Can you work these out from the model? Positions are in its coordinate system, mm. Give positions to 0.01 mm unless a question says otherwise; leave off trailing zeros. Write each loop counter-clockwise with the first axis right and the second up, starting at its lowest first coordinate (ties: lowest second). Pieces come first, ordered by that corner, then holes.
from build123d import *

# Parameters (mm, degrees)
SKIZZE1_W                                            = 180
SKIZZE1_H                                            = 65
AUFSATZ_LINEAR_AUSTRAGEN1_DEPTH                      = 5
STIRNSENKUNG_F_R_M3_ZYLINDERSCHRAUBE_MIT_D           = 3.6
STIRNSENKUNG_F_R_M3_ZYLINDERSCHRAUBE_MIT_DEPTH       = 9.1
STIRNSENKUNG_F_R_M3_ZYLINDERSCHRAUBE_MIT_CBORE_D     = 6.5
STIRNSENKUNG_F_R_M3_ZYLINDERSCHRAUBE_MIT_CBORE_DEPTH = 3.4
STIRNSENKUNG_F_R_M3_ZYLINDERSCHRAUBE_MIT_TIP         = 1.081549114
SCHNITT_LINEAR_AUSTRAGEN1_DEPTH                      = 66
SKIZZE7_R                                            = 6.5
SCHNITT_LINEAR_AUSTRAGEN2_DEPTH                      = 6.0000001


with BuildPart() as part:
    # Skizze1 → Aufsatz-Linear austragen1 (new body)
    with BuildSketch(Plane.XY):
        Rectangle(SKIZZE1_W, SKIZZE1_H)
    extrude(amount=AUFSATZ_LINEAR_AUSTRAGEN1_DEPTH)

    # Stirnsenkung für M3 Zylinderschraube mit Innensechskant1
    with Locations(Plane.XY.offset(5)):
        with Locations((-84, 0), (84, 0)):
            CounterBoreHole(STIRNSENKUNG_F_R_M3_ZYLINDERSCHRAUBE_MIT_D / 2, STIRNSENKUNG_F_R_M3_ZYLINDERSCHRAUBE_MIT_CBORE_D / 2, STIRNSENKUNG_F_R_M3_ZYLINDERSCHRAUBE_MIT_CBORE_DEPTH, depth=STIRNSENKUNG_F_R_M3_ZYLINDERSCHRAUBE_MIT_DEPTH)
            with Locations((0, 0, -(STIRNSENKUNG_F_R_M3_ZYLINDERSCHRAUBE_MIT_DEPTH + STIRNSENKUNG_F_R_M3_ZYLINDERSCHRAUBE_MIT_TIP / 2))):  # 118° drill point
                Cone(0, STIRNSENKUNG_F_R_M3_ZYLINDERSCHRAUBE_MIT_D / 2, STIRNSENKUNG_F_R_M3_ZYLINDERSCHRAUBE_MIT_TIP, mode=Mode.SUBTRACT)

    # Skizze6 → Schnitt-Linear austragen1 (cut, through all)
    with BuildSketch(Plane(origin=(0, 32.5, 0), x_dir=(1, 0, 0), z_dir=(0, 1, 0))):
        with BuildLine():
            Line((-90, -5), (-90, 5))
            ThreePointArc((-90, 5), (-87.071067812, -2.071067812), (-80, -5))
            Line((-80, -5), (-90, -5))
        make_face()
        with BuildLine():
            Line((80, -5), (90, -5))
            Line((90, -5), (90, 5))
            ThreePointArc((90, 5), (87.071067812, -2.071067812), (80, -5))
        make_face()
    extrude(amount=-SCHNITT_LINEAR_AUSTRAGEN1_DEPTH, mode=Mode.SUBTRACT)

    # Skizze7 → Schnitt-Linear austragen2 (cut, through all)
    with BuildSketch(Plane.XY.offset(5)):
        with Locations((65, -22.5)):
            Circle(SKIZZE7_R)
    extrude(amount=-SCHNITT_LINEAR_AUSTRAGEN2_DEPTH, mode=Mode.SUBTRACT)


solid = part.part
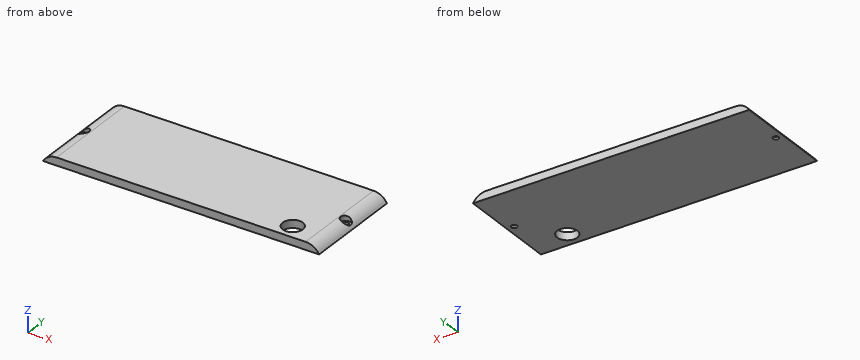
(1) Imagine slicing it at A-A, the plane y = -22.5. Write out the boundary of the cut face in (x, z).
Returned:
outline: (-88.66, 0) - (58.5, 0) - (58.5, 5) - (-80, 5) arc R10 ccw to start; (71.5, 0) - (88.66, 0) arc R10 ccw to (80, 5) - (71.5, 5) - close
(2) Will this pin go through, and if not, where does the flat tip stop? P1, Ø4, axis at x = -84, y = 0, coming from the +Z side.
Returned:
P1: stops at z = 1.6
(3) Imagine slicing it at D-D, the plane y = 0. Write out the boundary of the cut face in (x, z), plus the area to 3 significant figures.
Returned:
outline: (-88.66, 0) - (-85.8, 0) - (-85.8, 1.6) - (-87.25, 1.6) - (-87.25, 1.89) arc R10 ccw to start; (-82.2, 0) - (82.2, 0) - (82.2, 1.6) - (80.75, 1.6) - (80.75, 4.97) arc R10 ccw to (80, 5) - (-80, 5) arc R10 ccw to (-80.75, 4.97) - (-80.75, 1.6) - (-82.2, 1.6) - close; (85.8, 0) - (88.66, 0) arc R10 ccw to (87.25, 1.89) - (87.25, 1.6) - (85.8, 1.6) - close
area: 820 mm2
(4) If I drill on L1, parallel to Y at x = 84, z = 1.05; L2, parallel to Y at x = 65, z = 2.45; L3, parallel to X at y = -24, z = 2.6, over which ranges is the centre line in solid material (lowest first)?
Returned:
L1: y = -32.5 to -1.8, 1.8 to 32.5
L2: y = -32.5 to -29, -16 to 32.5
L3: x = -86.5 to 58.68, 71.32 to 86.5
(5) Imagine slicing it at C-C, the plane z = 2.8. Write out the boundary of the cut face in (x, y).
Returned:
outline: (-86.26, -32.5) - (86.26, -32.5) - (86.26, -2.34) arc R3.25 cw (long way) to (86.26, 2.34) - (86.26, 32.5) - (-86.26, 32.5) - (-86.26, 2.34) arc R3.25 cw (long way) to (-86.26, -2.34) - close; hole circle Ø13 at (65, -22.5)
(6) Imagine slicing it at B-B, the plane x = 65. Write out the boundary of the cut face in (y, z), plus the area to 3 significant figures.
Returned:
outline: (-32.5, 0) - (-29, 0) - (-29, 5) - (-32.5, 5) - close; (-16, 0) - (32.5, 0) - (32.5, 5) - (-16, 5) - close
area: 260 mm2
